Input: part model. Units: mm. Frame: model coordinates. A direction names the side the tool comes from. Coordinates: 2 decimals unless noted, no trailing zeros. Order: outer loops, then holes, each group sorted by start corner. A loop starts at its lowest first (then second) coordinate and runs counter-clockwise, first axis right, second up. Notation, with made-up numbers: (15.25, 63) - (65.25, 63) arc R10 ccw to (65.25, 73) - close; hole circle Ø6 at (-36, -2). An arc over 180 degrees is marked (long way). One line per question, with ' | ' between items. Start each with the question number.
```python
from build123d import *

# Parameters (mm, degrees)
SKETCH1_W                               = 50
SKETCH1_H                               = 50
BOSS_EXTRUDE1_DEPTH                     = 10
SKETCH2_W                               = 20
SKETCH2_H                               = 10
BOSS_EXTRUDE2_DEPTH                     = 30
SKETCH3_R                               = 10
BOSS_EXTRUDE3_DEPTH                     = 20
CBORE_FOR_M5_HEX_HEAD_BOLT1_D           = 5.5
CBORE_FOR_M5_HEX_HEAD_BOLT1_CBORE_D     = 12.24
CBORE_FOR_M5_HEX_HEAD_BOLT1_CBORE_DEPTH = 3.58
F_4_0MM_DOWEL_HOLE1_D                   = 4
CHAMFER1_SIZE                           = 10
FILLET1_R                               = 3


with BuildPart() as part:
    # Sketch1 → Boss-Extrude1 (new body)
    with BuildSketch(Plane(origin=(0, 0, 0), x_dir=(1, 0, 0), z_dir=(0, 1, 0))):
        with Locations((25, -25)):
            Rectangle(SKETCH1_W, SKETCH1_H)
    extrude(amount=BOSS_EXTRUDE1_DEPTH)

    # Sketch2 → Boss-Extrude2 (add)
    with BuildSketch(Plane(origin=(0, 10, 0), x_dir=(1, 0, 0), z_dir=(0, 1, 0))):
        with Locations((25, -10)):
            Rectangle(SKETCH2_W, SKETCH2_H)
    extrude(amount=BOSS_EXTRUDE2_DEPTH)

    # Sketch3 → Boss-Extrude3 (add)
    with BuildSketch(Plane(origin=(0, 0, 5), x_dir=(-1, 0, 0), z_dir=(0, 0, -1))):
        with Locations((-25, 40)):
            Circle(SKETCH3_R)
    extrude(amount=-BOSS_EXTRUDE3_DEPTH)

    # CBORE for M5 Hex Head Bolt1 (through all)
    with Locations(Plane.XY.offset(25)):
        with Locations((25, 40)):
            CounterBoreHole(CBORE_FOR_M5_HEX_HEAD_BOLT1_D / 2, CBORE_FOR_M5_HEX_HEAD_BOLT1_CBORE_D / 2, CBORE_FOR_M5_HEX_HEAD_BOLT1_CBORE_DEPTH)

    # Ø4.0mm Dowel Hole1 (through all)
    with Locations(Plane(origin=(0, 10, 0), x_dir=(1, 0, 0), z_dir=(0, 1, 0))):
        with Locations((12, -38), (38, -38)):
            Hole(F_4_0MM_DOWEL_HOLE1_D / 2)

    # Chamfer1
    chamfer1_edges = [part.edges().sort_by_distance(p)[0] for p in [
        (50, 5, 50),
        (0, 5, 50),
    ]]
    chamfer(chamfer1_edges, length=CHAMFER1_SIZE)

    # Fillet1
    fillet1_edges = [part.edges().sort_by_distance(p)[0] for p in [
        (25, 10, 0),
        (0, 10, 20),
        (50, 10, 20),
        (25, 10, 50),
        (5, 10, 45),
        (45, 10, 45),
    ]]
    fillet(fillet1_edges, radius=FILLET1_R)


solid = part.part
```
(1) Section A-A (z = 19). Output: boundary loops of the cut face in (x, y).
(2) Section C-C (x = 12). Output: boundary loops of the cut face in (y, z), then the cut area to 3 significant figures.
(3) Pin query (flat end, axial travel): pin 1 (6 mm diameter, centred on y = 17.5, z = 11.5, fed in from -X); pin 2 (22 mm diameter, centred on x = 25.5, y = 40.5, fed in from +Z); pin 3 (3 mm diameter, centred on x = 15.5, z = 34.5, fed in from +Y); pin 4 (4 mm diameter, centred on y = 13.5, z = 45, fed in from +X). Return the tip coordinate at first contact, or that it passes through.
(4) Material intervals for line 1 along X through (y, z) = (4, 38); line 2 along Y through (x, z) = (25, 24.35); line 3 along Z through (x, y) = (12, 7), sorted ascending. Write a range as from..to.
(5) Draft query along Z for faces 1 (the face through (5.708, 9.145, 44.432)), 2 (the face through (38, 5, 40)), 3 (the face through (49.1, 9.14, 19.72)). Return one class per face: +Z half, -Z half, draft (parallel to the pull), parting line (faces both ways), or undercut.
(6) Section B-B (z = 38). Output: boundary loops of the cut face in (x, y).
(7) Reachability of faces 4 (the face through (26, 37, 21.42)), 5 (the face through (15, 25, 10)), 6 (the face through (35, 25, 10)) from +Z, -Z, +X, -X, +Y, -Y: full face, straight path, thin tool, end or side. Return the list, or none.
(8) Section D-D (y = 4.5). Output: boundary loops of the cut face in (x, z).
Worked answers:
1) outline: (0, 0) - (50, 0) - (50, 7) arc R3 ccw to (47, 10) - (3, 10) arc R3 ccw to (0, 7) - close; circle Ø20 at (25, 40); hole circle Ø5.5 at (25, 40)
2) outline: (0, 0) - (7, 0) arc R3 ccw to (10, 3) - (10, 36) - (0, 36) - close; (0, 40) - (10, 40) - (10, 47) arc R3 ccw to (7, 50) - (0, 50) - close | area: 456 mm²
3) pin 1: stops at x = 15 | pin 2: stops at z = 25 | pin 3: stops at y = 10 | pin 4: passes through
4) line 1: x = 0..10, 14..36, 40..50 | line 2: y = 0..10, 30..33.88, 46.12..50 | line 3: z = 0..36, 40..50
5) face 1: +Z half | face 2: undercut | face 3: draft
6) outline: (0, 0) - (10, 0) - (10, 10) - (3, 10) arc R3 ccw to (0, 7) - close; (14, 0) - (36, 0) - (36, 10) - (14, 10) - close; (40, 0) - (50, 0) - (50, 7) arc R3 ccw to (47, 10) - (40, 10) - close
7) face 4: +Z | face 5: +Z, -Z, -X, +Y | face 6: +Z, -Z, +X, +Y
8) outline: (0, 0) - (50, 0) - (50, 40) - (40, 50) - (10, 50) - (0, 40) - close; hole circle Ø4 at (12, 38); hole circle Ø4 at (38, 38)
